For this review, take the finished solid that the model builds, in its own axes (mm). Face numbers are marked on the shaded views. A direction names the side the tool comes from. Give positions to 0.01 mm unless a question says otherwise; leave off trailing zeros. Order: outer loops, then holes, each group sorted by start corner. A loop starts at its lowest first (then second) coordinate and runs counter-clockwise, first axis right, second up.
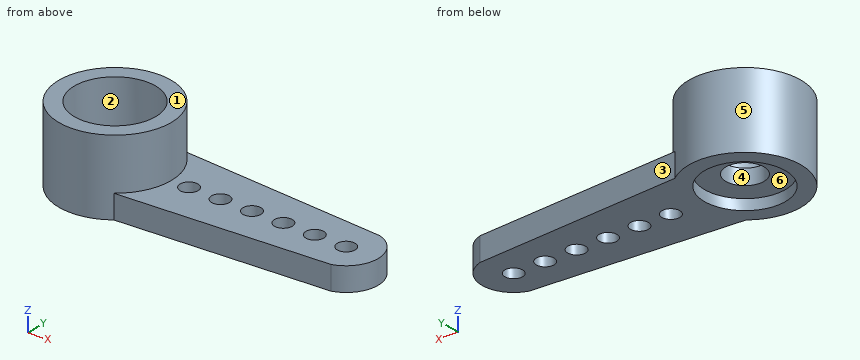
Autodesk Inventor part; units mm, degrees
ref_plane "YZ Plane" through (0, 0, 0) normal (1, 0, 0) x (0, 1, 0)
ref_plane "XZ Plane" through (0, 0, 0) normal (0, 1, 0) x (-1, 0, 0)
ref_plane "XY Plane" through (0, 0, 0) normal (0, 0, 1) x (1, 0, 0)
sketch "Sketch1" plane through (0, 0, 0) normal (0, 0, 1) x (1, 0, 0)
  circle A0 centre (0, 0) radius 3.45
  line L0 (0, 0) -> (14.75, 0) construction
  line L1 (14.75, 0) -> (14.75, 1.875) construction
  line L2 (14.75, 0) -> (14.75, -1.875) construction
  line L3 (14.75, 0) -> (16.15, 0) construction
  arc A1 (14.75, -1.875) -> (14.75, 1.875) centre (14.1944, 0) ccw
  line L4 (2.1159, 2.725) -> (2.1159, -2.725) construction
  line L5 (2.1159, 2.725) -> (14.75, 1.875)
  line L6 (2.1159, -2.725) -> (14.75, -1.875)
  circle A2 centre (14.1944, 0) radius 0.55
  circle A3 centre (4.5454, 0) radius 0.55
  circle A4 centre (6.4752, 0) radius 0.55
  circle A5 centre (8.405, 0) radius 0.55
  circle A6 centre (10.3348, 0) radius 0.55
  circle A7 centre (12.2646, 0) radius 0.55
  dimension "d0" = 6.9
  dimension "d1" = 14.75
  dimension "d2" = 1.875
  dimension "d3" = 1.875
  dimension "d4" = 1.4
  dimension "d5" = 5.45
  dimension "d12" = 1.1
  dimension "d13" = 1.1
  dimension "d14" = 1.1
  dimension "d15" = 1.1
  dimension "d16" = 1.1
  dimension "d17" = 1.1
  dimension "d18" = 1.9298
  dimension "d19" = 1.9298
  dimension "d20" = 1.9298
  dimension "d21" = 1.9298
  dimension "d22" = 1.9298
extrude "Extrusion1" add sketch "Sketch1" along normal blind 1.45 contours A0 L5 A1 L6
extrude "Extrusion2" add sketch "Sketch1" along normal blind 4.6 contours A0
sketch "Sketch2" plane through (0, 0, 0) normal (0, 0, -1) x (-1, 0, 0)
  arc A0 (-2.1159, -2.725) -> (-2.1159, 2.725) centre (0, 0) ccw
  circle A1 centre (0, 0) radius 1.175
  dimension "d27" = 2.35
extrude "Extrusion3" cut sketch "Sketch2" against normal up to next
sketch "Sketch3" plane through (0, 0, 4.6) normal (0, 0, 1) x (1, 0, 0)
  circle A0 centre (0, 0) radius 1.175
  circle A1 centre (0, 0) radius 3.45
  circle A2 centre (0, 0) radius 2.5
  dimension "d30" = 5
extrude "Extrusion4" cut sketch "Sketch3" against normal blind 3 contours A2
sketch "Sketch4" plane through (0, 0, 0) normal (0, 0, -1) x (-1, 0, 0)
  circle A0 centre (0, 0) radius 1.175
  circle A1 centre (0, 0) radius 2.5
  circle A2 centre (0, 0) radius 2.5
  circle A3 centre (0, 0) radius 2.5
extrude "Extrusion5" cut sketch "Sketch4" against normal blind 0.65
properties part number "Servo_Arm"
1) We need section D-D on y = 0. Count the separate pieces of the cut face and the enclosed holes in it, then the cut area to 3 significant figures.
Answer sheet:
separate pieces: 8
enclosed holes: 0
area: 20.1 mm2
2) Tool access review of the marked faces 1 and 2: name each direction out of +Z, -Z, +X, -X, +Y, -Y from which nothing blocks a thin tool from reaching the whole face with its end or side.
Answer sheet:
face 1: +Z, +X, -X, +Y, -Y
face 2: +Z
3) We need section C-C on z = 3.95. Give the boundary of the cut face in (x, y).
Answer sheet:
outline: circle Ø6.9 at (0, 0); hole circle Ø5 at (0, 0)
4) Clearance check with flat-ended pins moving along their axes: pin 1 (4 mm diameter, centred on x = -0.5, y = 1, fed in from +Z); pin 2 (2 mm diameter, centred on x = 6.5, z = 1.5, fed in from +Y); pin 3 (1.5 mm diameter, centred on y = 2, z = 4, fed in from +X); pin 4 (3 mm diameter, centred on x = 0, y = 0, fed in from -Z). State where each tip first meets the part, or that it passes through.
Answer sheet:
pin 1: stops at z = 4.6
pin 2: stops at y = 2.5
pin 3: stops at x = 3.22
pin 4: stops at z = 0.65
5) Draft analysis for pull direction X (two halves, no side actions). For the marked faces 3, 4, 5 and 6, state which applies: +X half, -X half, draft (parallel to the pull), parting line (faces both ways), or undercut.
Answer sheet:
face 3: +X half
face 4: undercut
face 5: parting line
face 6: undercut
6) To check wall thickness, follow line 1 (Y direction, x = 0, z = 2.4); line 2 (Y direction, x = 0, z = 0.95) (3 decimals); line 3 (Z direction, x = 8, y = 1). State the ranges of each line that lie inside material, in increasing order.
Answer sheet:
line 1: y = -3.45 to -2.5, 2.5 to 3.45
line 2: y = -3.45 to -1.175, 1.175 to 3.45
line 3: z = 0 to 1.45
7) We need section B-B on y = 1. Give the boundary of the cut face in (x, z), then the cut area to 3 significant figures.
Answer sheet:
outline: (-3.3, 0) - (-2.29, 0) - (-2.29, 0.65) - (-0.62, 0.65) - (-0.62, 1.6) - (-2.29, 1.6) - (-2.29, 4.6) - (-3.3, 4.6) - close; (0.62, 0.65) - (2.29, 0.65) - (2.29, 0) - (15.87, 0) - (15.87, 1.45) - (3.3, 1.45) - (3.3, 4.6) - (2.29, 4.6) - (2.29, 1.6) - (0.62, 1.6) - close
area: 30.7 mm2
8) We need section A-A on x = 0. Give the boundary of the cut face in (y, z) (3 decimals), then the cut area to 3 significant figures.
Answer sheet:
outline: (-3.45, 0) - (-2.5, 0) - (-2.5, 0.65) - (-1.175, 0.65) - (-1.175, 1.6) - (-2.5, 1.6) - (-2.5, 4.6) - (-3.45, 4.6) - close; (1.175, 0.65) - (2.5, 0.65) - (2.5, 0) - (3.45, 0) - (3.45, 4.6) - (2.5, 4.6) - (2.5, 1.6) - (1.175, 1.6) - close
area: 11.3 mm2
